Could you check a few things on this model? Use its own coordinates, in mm. Give positions to 0.01 mm unless a question says otherwise; leave off trailing zeros. Write each loop counter-clockwise with the first axis right and the second up, starting at its lowest first coordinate (ties: lowest second). Pieces come first, ordered by that corner, then holes. Notation, with made-up numbers: (75, -16) - (128, -16) arc R9 ccw to (128, -12) - close; hole circle Ø9 at (31, 4.5). An arc over 180 degrees is marked (long way). Answer in a Markdown table with one row per item.
from build123d import *

# Parameters (mm, degrees)
SALIENTE_EXTRUIR1_DEPTH = 3
CROQUIS1_R              = 1.55
CORTAR_EXTRUIR1_DEPTH   = 10


with BuildPart() as part:
    # Model → Saliente-Extruir1 (new body)
    with BuildSketch(Plane.XY):
        Polygon((186, 103), (186, 90.195), (183, 90.195), (183, 65.805), (186, 65.805), (186, 53), (220.805, 53), (220.805, 56), (245.195, 56), (245.195, 53), (269.585, 53), (280, 53), (280, 65.805), (283, 65.805), (283, 90.195), (280, 90.195), (280, 103), align=None)
    extrude(amount=SALIENTE_EXTRUIR1_DEPTH)

    # Croquis1 → Cortar-Extruir1 (cut)
    with BuildSketch(Plane.XY.offset(3)):
        with Locations((233, 78)):
            Circle(CROQUIS1_R)
        with Locations((198, 78)):
            Circle(CROQUIS1_R)
        with Locations((268, 78)):
            Circle(CROQUIS1_R)
    extrude(amount=-CORTAR_EXTRUIR1_DEPTH, mode=Mode.SUBTRACT)


solid = part.part
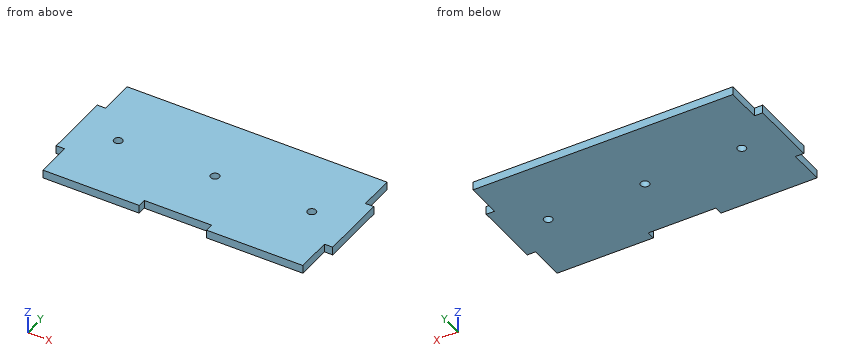
1) Imagine slicing it at B-B (y = 78). List the corners of the cut face in (x, z) for me.
Check values:
| item | result |
|---|---|
| outline | (183, 0) - (196.45, 0) - (196.45, 3) - (183, 3) - close; (199.55, 0) - (231.45, 0) - (231.45, 3) - (199.55, 3) - close; (234.55, 0) - (266.45, 0) - (266.45, 3) - (234.55, 3) - close; (269.55, 0) - (283, 0) - (283, 3) - (269.55, 3) - close |
2) Imagine slicing it at A-A (x = 233). List the corners of the cut face in (y, z) for me, then the cut area to 3 significant figures.
Check values:
| item | result |
|---|---|
| outline | (56, 0) - (76.45, 0) - (76.45, 3) - (56, 3) - close; (79.55, 0) - (103, 0) - (103, 3) - (79.55, 3) - close |
| area | 132 mm2 |
3) If I drill on line 1 (X direction, y = 78, z = 1.1); line 2 (Y direction, x = 268, z = 1.05); line 3 (Y direction, x = 233, z = 1.55), over which ranges is the centre line in solid material (lowest first)?
Check values:
| item | result |
|---|---|
| line 1 | x = 183 to 196.45, 199.55 to 231.45, 234.55 to 266.45, 269.55 to 283 |
| line 2 | y = 53 to 76.45, 79.55 to 103 |
| line 3 | y = 56 to 76.45, 79.55 to 103 |
4) Imagine slicing it at C-C (z = 0.45). List the corners of the cut face in (x, y) for me (3 decimals), then the cut area to 3 significant figures.
Check values:
| item | result |
|---|---|
| outline | (183, 65.805) - (186, 65.805) - (186, 53) - (220.805, 53) - (220.805, 56) - (245.195, 56) - (245.195, 53) - (280, 53) - (280, 65.805) - (283, 65.805) - (283, 90.195) - (280, 90.195) - (280, 103) - (186, 103) - (186, 90.195) - (183, 90.195) - close; hole circle Ø3.1 at (198, 78); hole circle Ø3.1 at (233, 78); hole circle Ø3.1 at (268, 78) |
| area | 4,750 mm2 |
5) Will these pins go through, and if not, where does the flat tip stop? P1, Ø1, axis at x = 238.5, z = 1, coming from the -Y side; P2, Ø1.5, axis at x = 281.5, z = 1, coming from the -Y side (3 decimals); P3, Ø0.9, axis at x = 184, z = 1, coming from the +Y side (3 decimals).
Check values:
| item | result |
|---|---|
| P1 | stops at y = 56 |
| P2 | stops at y = 65.805 |
| P3 | stops at y = 90.195 |
6) Imagine slicing it at D-D (x = 198). List the corners of the cut face in (y, z) for me.
Check values:
| item | result |
|---|---|
| outline | (53, 0) - (76.45, 0) - (76.45, 3) - (53, 3) - close; (79.55, 0) - (103, 0) - (103, 3) - (79.55, 3) - close |
